Build history of the part. All positions in model axes, mm. A direction names the side the tool comes from. Give positions to 0.01 mm unless a question says otherwise; leave off trailing zeros. Answer as a JSON object with one key per item and string values. Group by question number.
1. Drill centre lines: line 1 along X through (y, z) = (107, 9.5); line 2 along Z through (x, y) = (-138, 87.5); line 3 along Z through (x, y) = (-90.5, 10.5). Where is each one in solid material? Low to high. Write a range as [from, to].
2. Drop flat-ended pins along their axis: pin 1 Ø1 at (x, z) = (-41, 35) entering from +Y; pin 2 Ø8 at (x, y) = (-176, 129.5) entering from -Z; pin 3 Ø1 at (x, y) = (-14.5, 195) entering from +Z. Give the stop position or say it passes through.
3. Mould opens along Z. For faces 5 (the face through (0.875, 98.748, 60.088)), 6 (the face through (-195, 20, -14)), 7 (the face through (49.032, 100.678, 41.485)) say: released by +Z, released by -Z, zero draft, split by the parting line, or undercut.
4. 3-axis set-ups, long thin cutter, end or side, ignore diameter. For faces 1 (the face through (-37.962, 120.682, 32.293)), 2 (the face through (-62.5, 102, 30)), 3 (the face through (62.5, 102, 30)), 4 (the face through (0.875, 84.246, 27.496)): which of +Z, -Z, +X, -X, +Y, -Y reach the whole face in a straight line?
from build123d import *

# Parameters (mm, degrees)
EXTRUDE_START                                 = -25
EXTRUDE_PLATE_SHAPE_DEPTH                     = 50
CUT_EXTRUDE_ANGLE_DEPTH                       = 341.53226913
CUT_EXTRUDE_ANGLE_DEPTH_BACK                  = 341.53226913
CUT_EXTRUDE_SWITCH_HOLE_DEPTH                 = 340.963942654
CUT_EXTRUDE_SWITCH_HOLE_DEPTH_BACK            = 340.963942654
IGNITION_SWITCH_HOLE_R                        = 12.5
CUT_EXTRUDE_TOP_ENCLOSURE_HOLE_DEPTH          = 340.910991738
CUT_EXTRUDE_TOP_ENCLOSURE_HOLE_DEPTH_BACK     = 340.910991738
SKETCH23_R                                    = 2
CUT_EXTRUDE_BOTTOM_ENCLOSURE_HOLES_DEPTH      = 340.910991738
CUT_EXTRUDE_BOTTOM_ENCLOSURE_HOLES_DEPTH_BACK = 340.910991738
BOTTOM_ENCLOSURE_MOUNTING_HOLES_R             = 2
BOSS_EXTRUDE1_START                           = -6
SKETCH24_W                                    = 125
SKETCH24_H                                    = 75
BOSS_EXTRUDE1_DEPTH                           = 60
CUT_EXTRUDE_SHAFT_HOLE_DEPTH                  = 349.685760497
CUT_EXTRUDE_SHAFT_HOLE_DEPTH_BACK             = 349.685760497
STEERING_WHEEL_SHAFT_HOLE_R                   = 12.75
SKETCH26_W                                    = 456.008458956
SKETCH26_H                                    = 1.5
EXTRUDE_CUT_SLOT_DEPTH                        = 348.814796903
CUT_EXTRUDE17_DEPTH                           = 285.275916409
CUT_EXTRUDE17_DEPTH_BACK                      = 285.275916409
SKETCH28_R                                    = 4
CUT_EXTRUDE18_DEPTH                           = 351.351894744
CUT_EXTRUDE18_DEPTH_BACK                      = 60
SKETCH30_W                                    = 150
SKETCH30_H                                    = 50


# Read off the part's stored shape, not the designer's step: Extrude Plate Shape
with BuildPart() as part:
    # Extrude Plate Shape outline → Extrude Plate Shape (new body)
    with BuildSketch(Plane.XY.offset(EXTRUDE_START)):
        with BuildLine():
            Line((175, 0), (215.218833807, 40.218833807))
            ThreePointArc((215.218833807, 40.218833807), (226.057471223, 56.440000887), (229.863494748, 75.574172084))
            add(Edge.make_bspline(
                [(229.863494748, 75.574172084), (229.863497015, 220.574172084), (130.657195822, 208), (130.657198498, 108), (160, 250), (60, 250)],
                knots=[0, 0, 0, 0, 0, 0, 1, 1, 1, 1, 1, 1], degree=5))
            Line((60, 250), (-60, 250))
            add(Edge.make_bspline(
                [(-60, 250), (-160, 250), (-130.657198498, 108), (-130.657195822, 208), (-229.863497015, 220.574172084), (-229.863494748, 75.574172084)],
                knots=[0, 0, 0, 0, 0, 0, 1, 1, 1, 1, 1, 1], degree=5))
            ThreePointArc((-229.863494748, 75.574172084), (-226.057471223, 56.440000887), (-215.218833807, 40.218833807))
            Line((-215.218833807, 40.218833807), (-175, 0))
            Line((-175, 0), (175, 0))
        make_face()
    extrude(amount=EXTRUDE_PLATE_SHAPE_DEPTH)

    # 5-Degree Front Plate → Cut-Extrude Angle (cut, two sides: drawn at the far end of the back side and taken through both)
    with BuildSketch(Plane(origin=(0, 0, 0), x_dir=(0, 0, -1), z_dir=(1, 0, 0)).offset(-CUT_EXTRUDE_ANGLE_DEPTH_BACK)):
        Polygon((20.798974056, -10), (-14.747200293, 260), (35, 260), (35, -10), align=None)
        Polygon((-20.798974056, 260), (14.747200293, -10), (-35, -10), (-35, 260), align=None)
    extrude(amount=CUT_EXTRUDE_ANGLE_DEPTH + CUT_EXTRUDE_ANGLE_DEPTH_BACK, mode=Mode.SUBTRACT)

    # Ignition Switch Hole → Cut-Extrude Switch Hole (cut, two sides: drawn at the far end of the back side and taken through both)
    with BuildSketch(Plane(origin=(0, 2.521214434, -19.150524903), x_dir=(-1, 0, 0), z_dir=(0, 0.13052619222005532, -0.99144486137381)).offset(-CUT_EXTRUDE_SWITCH_HOLE_DEPTH_BACK)):
        with Locations(Location((150, 97.457030106, 0), (0, 0, 90))):
            Circle(IGNITION_SWITCH_HOLE_R)
    extrude(amount=CUT_EXTRUDE_SWITCH_HOLE_DEPTH + CUT_EXTRUDE_SWITCH_HOLE_DEPTH_BACK, mode=Mode.SUBTRACT)

    # Sketch23 → Cut-Extrude Top Enclosure Hole (cut, two sides: drawn at the far end of the back side and taken through both)
    with BuildSketch(Plane(origin=(0, 1.73805728, -13.201855735), x_dir=(1, 0, 0), z_dir=(0, -0.13052619222005535, 0.99144486137381)).offset(-CUT_EXTRUDE_TOP_ENCLOSURE_HOLE_DEPTH_BACK)):
        with Locations(Location((0, 236.854185237, 0), (0, 0, 270))):
            Circle(SKETCH23_R)
    extrude(amount=CUT_EXTRUDE_TOP_ENCLOSURE_HOLE_DEPTH + CUT_EXTRUDE_TOP_ENCLOSURE_HOLE_DEPTH_BACK, mode=Mode.SUBTRACT)

    # Bottom Enclosure Mounting Holes → Cut-Extrude Bottom Enclosure Holes (cut, two sides: drawn at the far end of the back side and taken through both)
    with BuildSketch(Plane(origin=(0, 1.73805728, -13.201855735), x_dir=(1, 0, 0), z_dir=(0, -0.13052619222005535, 0.99144486137381)).offset(-CUT_EXTRUDE_BOTTOM_ENCLOSURE_HOLES_DEPTH_BACK)):
        with Locations(Location((150, 11.746945092, 0), (0, 0, 270))):
            Circle(BOTTOM_ENCLOSURE_MOUNTING_HOLES_R)
        with Locations(Location((-150, 11.746945092, 0), (0, 0, 270))):
            Circle(BOTTOM_ENCLOSURE_MOUNTING_HOLES_R)
    extrude(amount=CUT_EXTRUDE_BOTTOM_ENCLOSURE_HOLES_DEPTH + CUT_EXTRUDE_BOTTOM_ENCLOSURE_HOLES_DEPTH_BACK, mode=Mode.SUBTRACT)

    # Sketch24 → Boss-Extrude1 (add)
    with BuildSketch(Plane(origin=(0, 2.521214434, -19.150524903), x_dir=(-1, 0, 0), z_dir=(0, 0.13052619222005538, -0.99144486137381)).offset(BOSS_EXTRUDE1_START)):
        with Locations((0, 124.614270251)):
            Rectangle(SKETCH24_W, SKETCH24_H)
    extrude(amount=-BOSS_EXTRUDE1_DEPTH)

    # Steering Wheel Shaft Hole → Cut-Extrude Shaft Hole (cut, two sides: drawn at the far end of the back side and taken through both)
    with BuildSketch(Plane(origin=(0, 2.521214434, -19.150524903), x_dir=(-1, 0, 0), z_dir=(0, 0.13052619222005532, -0.99144486137381)).offset(-CUT_EXTRUDE_SHAFT_HOLE_DEPTH_BACK)):
        with Locations(Location((0, 124.614270251, 0), (0, 0, 90))):
            Circle(STEERING_WHEEL_SHAFT_HOLE_R)
    extrude(amount=CUT_EXTRUDE_SHAFT_HOLE_DEPTH + CUT_EXTRUDE_SHAFT_HOLE_DEPTH_BACK, mode=Mode.SUBTRACT)

    # Sketch26 → Extrude-Cut Slot (cut, through all)
    with BuildSketch(Plane(origin=(0, 1.73805728, -13.201855735), x_dir=(1, 0, 0), z_dir=(0, -0.13052619222005535, 0.99144486137381))):
        with Locations((0, 124.614270251)):
            Rectangle(SKETCH26_W, SKETCH26_H)
    extrude(amount=EXTRUDE_CUT_SLOT_DEPTH, mode=Mode.SUBTRACT)

    # Sketch28 → Cut-Extrude17 (cut, two sides: drawn at the far end of the back side and taken through both)
    with BuildSketch(Plane(origin=(0, 160.727360196, 21.1601584), x_dir=(1, 0, 0), z_dir=(0, 0.99144486137381, 0.1305261922200554)).offset(-CUT_EXTRUDE17_DEPTH_BACK)):
        with Locations(Location((-47.5, -31.684225972, 0), (0, 0, 270))):
            Circle(SKETCH28_R)
        with Locations(Location((-47.5, -1.684225972, 0), (0, 0, 270))):
            Circle(SKETCH28_R)
        with Locations(Location((47.5, -31.684225972, 0), (0, 0, 90))):
            Circle(SKETCH28_R)
        with Locations(Location((47.5, -1.684225972, 0), (0, 0, 90))):
            Circle(SKETCH28_R)
    extrude(amount=CUT_EXTRUDE17_DEPTH + CUT_EXTRUDE17_DEPTH_BACK, mode=Mode.SUBTRACT)

    # Sketch30 → Cut-Extrude18 (cut, two sides: drawn at the far end of the back side and taken through both)
    with BuildSketch(Plane(origin=(0, -6.093514253, 46.284835948), x_dir=(1, 0, 0), z_dir=(0, -0.1305261922200554, 0.99144486137381)).offset(-CUT_EXTRUDE18_DEPTH_BACK)):
        with Locations((0, 149.614270251)):
            Rectangle(SKETCH30_W, SKETCH30_H)
    extrude(amount=CUT_EXTRUDE18_DEPTH + CUT_EXTRUDE18_DEPTH_BACK, mode=Mode.SUBTRACT)


solid = part.part
Established:
{
 "1": {"line 1": "x = [-62.5, 62.5]", "line 2": "z = [-7.96, -1.91]", "line 3": "z = [-18.1, -12.05]"},
 "2": {"pin 1": "stops at y = 120.39", "pin 2": "stops at z = -2.96", "pin 3": "stops at z = 12.31"},
 "3": {"face 5": "released by +Z", "face 6": "zero draft", "face 7": "undercut"},
 "4": {"face 1": "+Z, +X, -X", "face 2": "+Z, -X, -Y", "face 3": "+Z, +X, -Y", "face 4": "+X, -X, -Y"}
}
